from build123d import *

# Parameters (mm, degrees)
CYLINDER397_R          = 1.6
CYLINDER397_DEPTH      = 10
CYLINDER398_R          = 1.6
CYLINDER398_DEPTH      = 10
CYLINDER399_R          = 1.6
CYLINDER399_DEPTH      = 10
CYLINDER400_R          = 1.6
CYLINDER400_DEPTH      = 10
BOX271_W               = 15
BOX271_H               = 42
BOX271_DEPTH           = 20
BOX270_W               = 50
BOX270_H               = 82
BOX270_DEPTH           = 20
FILLET104_R            = 2
BOX268_W               = 58
BOX268_H               = 82
BOX268_DEPTH           = 10
BOX268_PLACEMENT_ANGLE = 3
BOX269_W               = 50
BOX269_H               = 82
BOX269_DEPTH           = 22
FILLET105_R            = 5


with BuildPart() as cylinder397:
    # Cylinder397 → Cylinder397 (new body)
    with BuildSketch(Plane(origin=(320, -4, -6), x_dir=(1, 0, 0), z_dir=(0, 0, 1))):
        Circle(CYLINDER397_R)
    extrude(amount=CYLINDER397_DEPTH)


with BuildPart() as fusion344:
    # Cylinder398 → Cylinder398 (new body)
    with BuildSketch(Plane(origin=(320, 66, -6), x_dir=(1, 0, 0), z_dir=(0, 0, 1))):
        Circle(CYLINDER398_R)
    extrude(amount=CYLINDER398_DEPTH)

    # Fusion344: union Cylinder397
    add(cylinder397.part)


with BuildPart() as fusion344_1:
    # Fusion344 placement: moved
    add(fusion344.part.moved(Location((2, 0, 0))))


with BuildPart() as cylinder399:
    # Cylinder399 → Cylinder399 (new body)
    with BuildSketch(Plane(origin=(320, -4, -6), x_dir=(1, 0, 0), z_dir=(0, 0, 1))):
        Circle(CYLINDER399_R)
    extrude(amount=CYLINDER399_DEPTH)


with BuildPart() as fusion346:
    # Cylinder400 → Cylinder400 (new body)
    with BuildSketch(Plane(origin=(320, 66, -6), x_dir=(1, 0, 0), z_dir=(0, 0, 1))):
        Circle(CYLINDER400_R)
    extrude(amount=CYLINDER400_DEPTH)

    # Fusion345: union Cylinder399
    add(cylinder399.part)


with BuildPart() as fusion346_1:
    # Fusion345 placement: moved
    add(fusion346.part.moved(Location((33, 0, 0))))

    # Fusion346: union Fusion344
    add(fusion344_1.part)


with BuildPart() as cube351:
    # Box271 → Box271 (new body)
    with BuildSketch(Plane(origin=(312.5, 10, -5), x_dir=(1, 0, 0), z_dir=(0, 0, 1))):
        with Locations((7.5, 21)):
            Rectangle(BOX271_W, BOX271_H)
    extrude(amount=BOX271_DEPTH)


with BuildPart() as fillet104:
    # Box270 → Box270 (new body)
    with BuildSketch(Plane(origin=(312.5, 0, 0), x_dir=(1, 0, 0), z_dir=(0, 0, 1))):
        with Locations((25, 41)):
            Rectangle(BOX270_W, BOX270_H)
    extrude(amount=BOX270_DEPTH)

    # Fillet104
    fillet104_edges = [fillet104.edges().sort_by_distance(p)[0] for p in [
        (337.5, 0, 0),
        (337.5, 82, 0),
    ]]
    fillet(fillet104_edges, radius=FILLET104_R)


with BuildPart() as fillet104_1:
    # Fillet104 placement: moved
    add(fillet104.part.moved(Location((0, -10, 0))))


with BuildPart() as cube348:
    # Box268 → Box268 (new body)
    with BuildSketch(Plane.XY):
        with Locations((29, 41)):
            Rectangle(BOX268_W, BOX268_H)
    extrude(amount=BOX268_DEPTH)


with BuildPart() as cube348_1:
    # Box268 placement: moved
    add(cube348.part.moved(Location((308.5, -10, -14.5))).rotate(Axis((308.5, -10, -14.5), (0, -1, 0)), BOX268_PLACEMENT_ANGLE))


with BuildPart() as battery_box_holder_wide:
    # Box269 → Box269 (new body)
    with BuildSketch(Plane(origin=(312.5, -10, -5), x_dir=(1, 0, 0), z_dir=(0, 0, 1))):
        with Locations((25, 41)):
            Rectangle(BOX269_W, BOX269_H)
    extrude(amount=BOX269_DEPTH)

    # Cut281: cut Cube348
    add(cube348_1.part, mode=Mode.SUBTRACT)

    # Cut282: cut Fillet104
    add(fillet104_1.part, mode=Mode.SUBTRACT)

    # Cut283: cut Cube351
    add(cube351.part, mode=Mode.SUBTRACT)

    # Cut284: cut Fusion346
    add(fusion346_1.part, mode=Mode.SUBTRACT)

    # Fillet105
    fillet105_edges = [battery_box_holder_wide.edges().sort_by_distance(p)[0] for p in [
        (312.5, 10, -2.138323),
        (327.5, 10, -1.745264),
        (327.5, 52, -1.745264),
        (312.5, 52, -2.138323),
    ]]
    fillet(fillet105_edges, radius=FILLET105_R)


solid = battery_box_holder_wide.part
Geometry check sheet. Reference: the model listing, model coordinates, mm. A direction names the side the tool comes from. Round coordinates to 2 decimals unless told otherwise and drop trailing zeros. Loops run counter-clockwise (first coordinate to the right, second up) from the corner with the lowest first, then second, coordinate; pieces in that order, holes last.
Item 1: Thickness scan on line 1 (Y direction, x = 322, z = -1.7); line 2 (X direction, y = 66, z = -0.65); line 3 (Y direction, x = 353, z = -1.65). Record the ranges inside material, lowest first.
Item 2: Access from +Z, -Z, +X, -X, +Y, -Y to the whole of each face (thin tool, end or side, straight path). Record for faces 1 (the flat face through (312.5, 64, -2)), 2 (the cylindrical face through (326.07, 50.5, -1.85)), 3 (the flat face through (343, 32, 0)).
Item 3: Cross-section at A-A on x = 353. Record the boundary of the cut face in (y, z).
Item 4: Mould release check, pull along X, two halves, no side actions. Record for faces 4 (the cylindrical face through (320.4, 66.07, -1.96)), 5 (the flat face through (337, 72, 0)), 6 (the cylindrical face through (314, 53.43, -2.11)): pulls with the +X half, pulls with the -X half, needs draft (parallel to the pull), parting line crosses it, or undercut.
Item 5: Cross-section at D-D on x = 334. Record the boundary of the cut face in (y, z).
Item 6: Gauge pin test, flat ends, axial feed: pin 1 (2 mm diameter, centred on y = 25, z = -0.5, fed in from -X); pin 2 (1.9 mm diameter, centred on x = 322, y = 66, fed in from +Z); pin 3 (5 mm diameter, centred on x = 322, y = -4, fed in from +Z); pin 4 (4 mm diameter, centred on x = 325.5, y = 1, fed in from -Z). Record the tip position at first contact, or that the pin passes through.
Item 7: Cross-section at C-C on y = 44.5. Record the boundary of the cut face in (x, z).
Item 8: Cross-section at B-B on y = -4. Record the boundary of the cut face in (x, z), then the cut area to 3 significant figures.
Answer sheet:
1. line 1: y = -10 to -5.6, -2.4 to 10, 52 to 64.4, 67.6 to 72
1. line 2: x = 312.5 to 320.4, 323.6 to 351.4, 354.6 to 362.5
1. line 3: y = -10 to -5.6, -2.4 to 64.4, 67.6 to 72
2. face 1: +Z, -Z, -X, +Y, -Y
2. face 2: +Z, -Z, -X
2. face 3: +Z, +X, -X
3. outline: (-10, -2.15) - (-5.6, -2.15) - (-5.6, 0) - (-8, 0) arc R2 cw to (-10, 2) - close; (-2.4, -2.15) - (64.4, -2.15) - (64.4, 0) - (-2.4, 0) - close; (67.6, -2.15) - (72, -2.15) - (72, 2) arc R2 cw to (70, 0) - (67.6, 0) - close
4. face 4: undercut
4. face 5: needs draft
4. face 6: pulls with the -X half
5. outline: (-10, -3.15) - (72, -3.15) - (72, 2) arc R2 cw to (70, 0) - (-8, 0) arc R2 cw to (-10, 2) - close
6. pin 1: stops at x = 327.5
6. pin 2: passes through
6. pin 3: stops at z = 0
6. pin 4: stops at z = -3.7
7. outline: (327.5, -3.49) - (362.5, -1.66) - (362.5, 0) - (327.5, 0) - close
8. outline: (312.5, -4.28) - (320.4, -3.86) - (320.4, 0) - (312.5, 0) - close; (323.6, -3.69) - (351.4, -2.24) - (351.4, 0) - (323.6, 0) - close; (354.6, -2.07) - (362.5, -1.66) - (362.5, 0) - (354.6, 0) - close
8. area: 129 mm2
